Autodesk Inventor part; units mm, degrees
ref_plane "YZ Plane" through (0, 0, 0) normal (1, 0, 0) x (0, 1, 0)
ref_plane "XZ Plane" through (0, 0, 0) normal (0, 1, 0) x (-1, 0, 0)
ref_plane "XY Plane" through (0, 0, 0) normal (0, 0, 1) x (1, 0, 0)
sketch "Sketch1" plane through (0, 0, 0) normal (0, 0, 1) x (1, 0, 0)
  circle A0 centre (0, 0) radius 11.5
  line L0 (5, -11.5) -> (37, -11.5)
  line L1 (37, -11.5) -> (37, -8)
  line L2 (37, -8) -> (5, -8)
  line L3 (5, -8) -> (5, -11.5)
  line L4 (37, -8) -> (37, -0.5)
  line L5 (37, -0.5) -> (10.3562, 5)
  line L6 (0, 0) -> (0, -11.5) construction
  line L7 (0, -11.5) -> (5, -11.5)
  dimension "d0" = 23
  dimension "d2" = 3.5
  dimension "d3" = 11
  dimension "d4" = 5
  dimension "d5" = 5
  dimension "d6" = 37
extrude "Extrusion1" add sketch "Sketch1" along normal mid plane 60
extrude "Extrusion2" cut sketch "Sketch1" along normal mid plane 54 contours A0 L2 L3 | A0 L5 L4 L2 | A0 L3 L7 picked at (-2.9713, 3.3704)
sketch "Sketch2" plane through (0, 0, 0) normal (0, 1, 0) x (-1, 0, 0)
  line L0 (0, 0) -> (-30, 0) construction
  arc A0 (-27.5, -2.5) -> (-32.5, -2.5) centre (-30, -2.5) ccw construction
  arc A1 (-32.5, 2.5) -> (-27.5, 2.5) centre (-30, 2.5) ccw construction
  line L1 (-32.5, -2.5) -> (-32.5, 2.5)
  line L2 (-27.5, -2.5) -> (-27.5, 2.5)
  line L3 (-30, -2.5) -> (-30, 2.5) construction
  arc A2 (-32.5, -2.5) -> (-27.5, -2.5) centre (-30, -2.5) ccw
  arc A3 (-27.5, 2.5) -> (-32.5, 2.5) centre (-30, 2.5) ccw
  line L4 (-22.5, -15) -> (-22.5, -10)
  line L5 (-17.5, -15) -> (-17.5, -10)
  arc A4 (-22.5, -15) -> (-17.5, -15) centre (-20, -15) ccw
  arc A5 (-17.5, -10) -> (-22.5, -10) centre (-20, -10) ccw
  line L6 (-20, -15) -> (-20, -10) construction
  arc A6 (-17.5, 15) -> (-22.5, 15) centre (-20, 15) ccw
  line L7 (-22.5, 15) -> (-22.5, 10)
  line L8 (-17.5, 15) -> (-17.5, 10)
  arc A7 (-22.5, 10) -> (-17.5, 10) centre (-20, 10) ccw
  line L9 (-20, 15) -> (-20, 10) construction
  line L10 (-17.5, -12.5) -> (-22.5, -12.5) construction
  line L11 (-17.5, 12.5) -> (-22.5, 12.5) construction
  dimension "d13" = 30
  dimension "d18" = 5
  dimension "d19" = 5
  dimension "d22" = 10
  dimension "d23" = 25
extrude "Extrusion3" cut sketch "Sketch2" against normal through all
fillet "Fillet1" radius 4 4 edges at (37, -0.5, -28.5) (37, -0.5, 28.5) (10.3562, 5, -28.5) (10.3562, 5, 28.5)
properties part number "carrier-end" material "ABS Plastic"
Can you work these out from the model? Positions are in its coordinate system, mm. A direction names the side the tool comes from. Give positions to 0.01 mm unless a question says otherwise; leave off trailing zeros. Order: outer loops, then holes, each group sorted by start corner. A loop starts at its lowest first (then second) coordinate and runs counter-clockwise, first axis right, second up. Notation, with made-up numbers: M 58,89 L 102,89 A16 ccw 102,100 Z; hole C 86.25,12 d8. An arc over 180 degrees is marked long. One line per question, with ' | ' between items.
Item 1: Please list where these lines run through material, in increasing order: L1, parallel to Z at x = 29.5, y = -3.25; L2, parallel to X at y = -9.5, z = -1; L3, parallel to Y at x = 30, z = -19.
Answer block:
L1: z = -30 to -27, 27 to 30 | L2: x = 5 to 27.5, 32.5 to 37 | L3: y = -11.5 to -8
Item 2: We'd pull the mould along X, two halves only. Please class faces 1 (the face through (-10.283, 5.149, -28.521)), 2 (the face through (36.077, -1.203, -28.521)), 3 (the face through (19.9, -9.7, 17.5)): released by +X, released by -X, zero draft, split by the parting line, or undercut.
Answer block:
face 1: split by the parting line | face 2: released by +X | face 3: undercut
Item 3: Suppose I cut it at B-B, the plane x = 20. Write out the boundary of the cut face in (y, z).
Answer block:
outline: M -11.5,-30 L 3.01,-30 L 3.01,-27 L -8,-27 L -8,-17.5 L -11.5,-17.5 Z; M -11.5,-7.5 L -8,-7.5 L -8,7.5 L -11.5,7.5 Z; M -11.5,17.5 L -8,17.5 L -8,27 L 3.01,27 L 3.01,30 L -11.5,30 Z
Item 4: Suppose I cut it at D-D, the plane y = -9. Write out the boundary of the cut face in (x, z), then the cut area to 3 significant figures.
Answer block:
outline: M -7.16,-30 L 37,-30 L 37,30 L -7.16,30 L -7.16,27 L 5,27 L 5,-27 L -7.16,-27 Z; hole M 17.5,-15 A2.5 ccw 22.5,-15 L 22.5,-10 A2.5 ccw 17.5,-10 Z; hole M 17.5,10 A2.5 ccw 22.5,10 L 22.5,15 A2.5 ccw 17.5,15 Z; hole M 27.5,-2.5 A2.5 ccw 32.5,-2.5 L 32.5,2.5 A2.5 ccw 27.5,2.5 Z | area: 1,860 mm2
Item 5: Suppose I cut it at A-A, the plane z = 1.5. Write out the boundary of the cut face in (x, y), then the cut area to 3 significant figures.
Answer block:
outline: M 5,-11.5 L 27.5,-11.5 L 27.5,-8 L 5,-8 Z; M 32.5,-11.5 L 37,-11.5 L 37,-8 L 32.5,-8 Z | area: 94.5 mm2
Item 6: I'm going to push flat-ended pins straight in: pin 1 Ø12 at (y, z) = (-0.5, -2.5) entering from -X; pin 2 Ø16 at (x, z) = (27.5, 13.5) entering from +Y; pin 3 Ø1 at (y, z) = (-10.5, -12) entering from -X. Where does each tip first touch, or does it pass through?
Answer block:
pin 1: passes through | pin 2: stops at y = -8 | pin 3: stops at x = 5
Item 7: Suppose I cut it at C-C, the plane x = -5. Write out the boundary of the cut face in (y, z).
Answer block:
outline: M -10.36,-30 L 10.36,-30 L 10.36,-27 L -10.36,-27 Z; M -10.36,27 L 10.36,27 L 10.36,30 L -10.36,30 Z
Item 8: For faces 4 (the face through (21, -8, 0)), 5 (the face through (5, -10, 0)), 6 (the face through (19.9, -9.7, -7.5)), which set-ups out of +Z, -Z, +X, -X, +Y, -Y let a thin tool reach every point of the face, with its end or its side?
Answer block:
face 4: +X, -X, +Y | face 5: -X, +Y, -Y | face 6: +Y, -Y
